```python
from build123d import *

# Parameters (mm, degrees)
SKETCH1_W           = 41
SKETCH1_H           = 4.788
SKETCH1_W_2         = 12
SKETCH1_H_2         = 3.175
BOSS_EXTRUDE1_DEPTH = 3.175
SKETCH2_W           = 7
SKETCH2_H           = 3.175
BOSS_EXTRUDE3_DEPTH = 3.175


with BuildPart() as part:
    # Sketch1 → Boss-Extrude1 (new body)
    with BuildSketch(Plane.XY):
        Rectangle(SKETCH1_W, SKETCH1_H)
        with Locations((-9.5, -3.9815)):
            Rectangle(SKETCH1_W_2, SKETCH1_H_2)
        with Locations((9.5, -3.9815)):
            Rectangle(SKETCH1_W_2, SKETCH1_H_2)
    extrude(amount=BOSS_EXTRUDE1_DEPTH)

    # Sketch2 → Boss-Extrude3 (add)
    with BuildSketch(Plane.XY.offset(3.175)):
        with Locations((0, -3.9815)):
            Rectangle(SKETCH2_W, SKETCH2_H)
    extrude(amount=-BOSS_EXTRUDE3_DEPTH)


solid = part.part
```
Design review of the part built by this model. Coordinates are the model's own, in mm. A direction names the side the tool comes from. Round coordinates to 2 decimals unless told otherwise and drop trailing zeros. Write each loop counter-clockwise with the first axis right and the second up, starting at its lowest first coordinate (ties: lowest second). Pieces come first, ordered by that corner, then holes. Notation, with made-up numbers: (36, 59.5) -> (68, 59.5) arc R9 cw to (68, 71.5) -> close; hole circle Ø5 at (21, 81.5). An arc over 180 degrees is marked (long way). Write item = value, one per line. Start each with the question number.
1) Take a section at C-C, the plane y = -4.25. State the section outline as (x, z) points (3 decimals), plus the area to 3 significant figures.
2) Tool access review of faces 1 (the face through (-15.5, -4, 2)), 2 (the face through (-20.5, 0, 2)), 3 (the face through (18, -2.394, 2)): name each direction out of +Z, -Z, +X, -X, +Y, -Y from which nothing blocks a thin tool from reaching the whole face with its end or side.
3) Clearance check with flat-ended pins moving along their axes: pin 1 (1.6 mm diameter, centred on y = -4.5, z = 2, fed in from -X); pin 2 (1 mm diameter, centred on y = -3, z = 1.5, fed in from +X). State where each tip first meets the part, or that it passes through.
4) Take a section at A-A, the plane z = 0.65. State the section outline as (x, y) points, plus the area to 3 significant figures.
5) Take a section at B-B, the plane x = 17. State the section outline as (y, z) points (3 decimals).
6) Wall thickness on probe 1 along X at (y, z) = (-2.75, 2); probe 2 along Y at (x, z) = (-18, 1.7): over which ranges is each line inside the solid? List them lowest first. Write a range as from..to.
Results list:
q1.outline = (-15.5, 0) -> (15.5, 0) -> (15.5, 3.175) -> (-15.5, 3.175) -> close
q1.area = 98.4 mm²
q2.face_1 = +Z, -Z, -X, -Y
q2.face_2 = +Z, -Z, -X, +Y, -Y
q2.face_3 = +Z, -Z, +X, -Y
q3.pin_1 = -15.5
q3.pin_2 = 15.5
q4.outline = (-20.5, -2.39) -> (-15.5, -2.39) -> (-15.5, -5.57) -> (15.5, -5.57) -> (15.5, -2.39) -> (20.5, -2.39) -> (20.5, 2.39) -> (-20.5, 2.39) -> close
q4.area = 295 mm²
q5.outline = (-2.394, 0) -> (2.394, 0) -> (2.394, 3.175) -> (-2.394, 3.175) -> close
q6.probe_1 = -15.5..15.5
q6.probe_2 = -2.39..2.39
